Source: three-view drawing plus pictorial views. Frame: mm from the lowest corner of the part. Give positions to 0.01 mm unless a question says otherwise; leave off trailing zeros. Loops run counter-clockwise (first coordinate to the right, second up) from the corner with the lowest first, then second, coordinate; pieces in that order, holes last. Notation, with made-up numbers: M 70,76.5 L 92,76.5 A25 ccw 92,103.5 Z; hole C 19,44.5 d5. An arc over 180 degrees is marked long. One line per item, written item: value. Start each with the question number.
(1) Ray query, line 1 along Y through (x, z) = (4, 1.5); line 2 along Z through (x, y) = (5.25, 4.5); line 3 along Y through (x, z) = (5.25, 0.5). Return the intervals inside material, ascending. Write a range as from..to.
(2) Section B-B on z = 4. Output: boundary loops of the cut face in (x, y), plus the area to 3 significant figures.
(3) Section A-A on z = 1.3. Output: boundary loops of the cut face in (x, y).
(4) Pin query (flat end, axial travel): P1, Ø1.8, axis at x = 3.5, y = 4, coming from the -Z side. Return the tip coordinate at first contact, or that it passes through.
(5) Pull-direction query (Y, two-part tool) for the marked faces 1, 2 and 3; classes: released by +Y, released by -Y, zero draft, split by the parting line, or undercut.
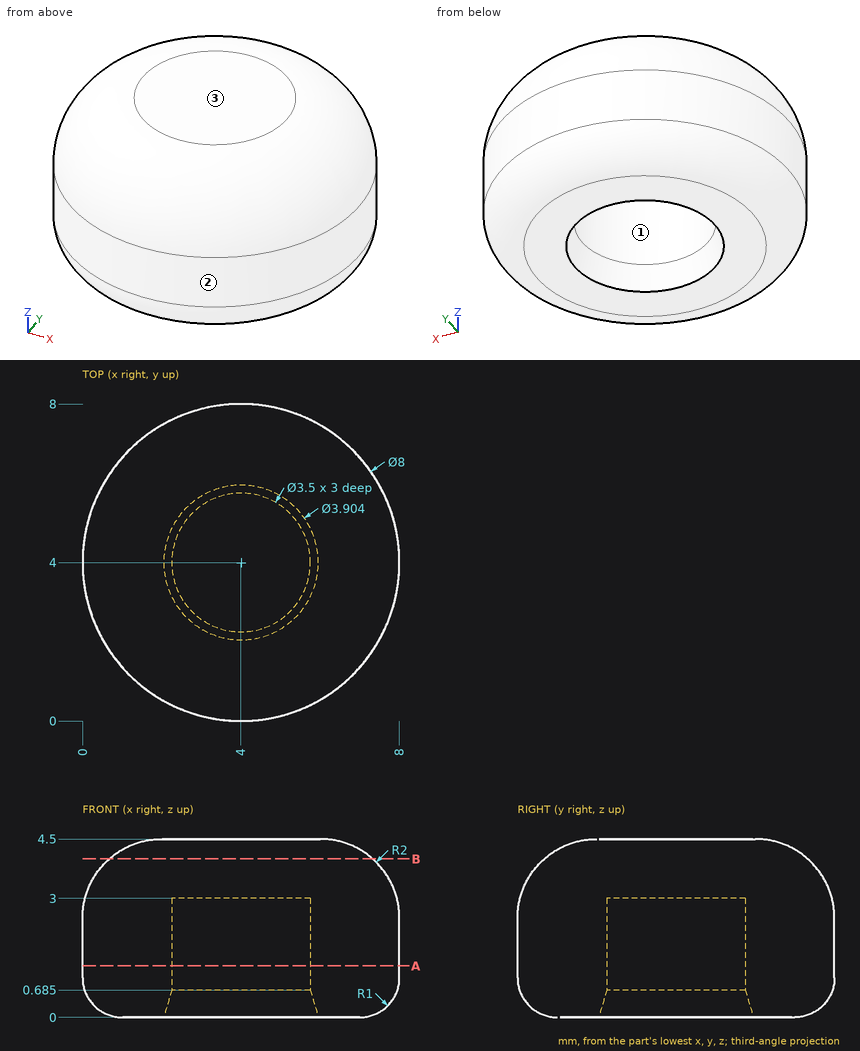
Output values:
1. line 1: y = 0..2.25, 5.75..8
1. line 2: z = 3..4.5
1. line 3: y = 0.34..2.7, 5.3..7.66
2. outline: C 4,4 d6.65
2. area: 34.7 mm²
3. outline: C 4,4 d8; hole C 4,4 d3.5
4. P1: stops at z = 3
5. face 1: undercut
5. face 2: split by the parting line
5. face 3: zero draft
